Here's the drawing with two shaded views (mm, measured from the low corner). I have some questions. Coordinates: 2 decimals unless noted, no trailing zeros. Loops run counter-clockwise (first coordinate to the right, second up) from the corner with the lowest first, then second, coordinate; pieces in that order, holes last. Notation, with made-up numbers: M -12,-24.5 L 11,-24.5 A20 cw 11,3.5 Z; hole C 8.25,18.5 d2. An arc over 180 degrees is marked long. Return JSON: item names as keys, results as strings. Group by question number.
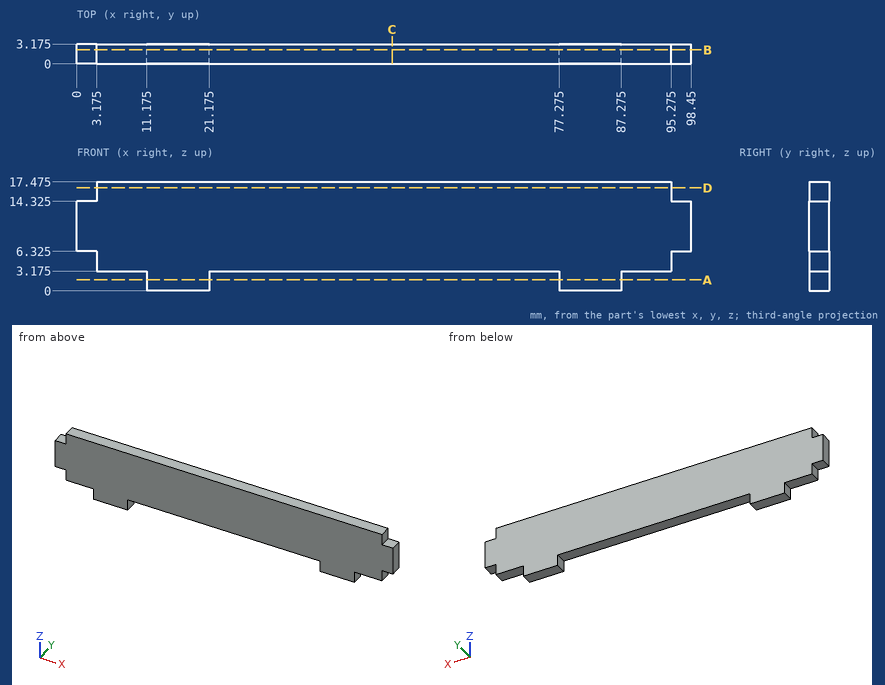
(1) Imagine slicing it at A-A, the plane z = 1.75. Write out the boundary of the cut face in (x, y) (3 decimals), then the cut area to 3 significant figures.
(2) Imagine slicing it at B-B, the plane y = 2.25. Write out the boundary of the cut face in (x, z) (3 decimals).
(3) Will these pins go through, and if not, where does the flat tip stop? P1, Ø1.6, axis at y = 1.5, z = 5, coming from the -X side (3 decimals); P2, Ø1, axis at y = 1, z = 1.5, coming from the +X side (3 decimals); P3, Ø1, axis at x = 69.5, y = 1, coming from the -Z side (3 decimals).
(4) Imagine slicing it at D-D, the plane z = 16.5. Write out the boundary of the cut face in (x, y) (3 decimals), then the cut area to 3 significant figures.
(5) If I drill on L1, parallel to X at y = 1.15, z = 2.25 (3 decimals); L2, parallel to Z at x = 71.5, y = 1.3 (3 decimals); L3, parallel to X at y = 1.65, z = 16 (3 decimals), over which ranges is the centre line in solid material (lowest first)? Write a range as [from, to].
(6) Imagine slicing it at C-C, the plane x = 50.5. Write out the boundary of the cut face in (y, z) (3 decimals).
Checks:
{
 "1": {"outline": "M 11.175,0 L 21.175,0 L 21.175,3.175 L 11.175,3.175 Z; M 77.275,0 L 87.275,0 L 87.275,3.175 L 77.275,3.175 Z", "area": "63.5 mm²"},
 "2": {"outline": "M 0,6.325 L 3.175,6.325 L 3.175,3.175 L 11.175,3.175 L 11.175,0 L 21.175,0 L 21.175,3.175 L 77.275,3.175 L 77.275,0 L 87.275,0 L 87.275,3.175 L 95.275,3.175 L 95.275,6.325 L 98.45,6.325 L 98.45,14.325 L 95.275,14.325 L 95.275,17.475 L 3.175,17.475 L 3.175,14.325 L 0,14.325 Z"},
 "3": {"P1": "x = 3.175", "P2": "x = 87.275", "P3": "z = 3.175"},
 "4": {"outline": "M 3.175,0 L 95.275,0 L 95.275,3.175 L 3.175,3.175 Z", "area": "292 mm²"},
 "5": {"L1": "[11.175, 21.175], [77.275, 87.275]", "L2": "[3.175, 17.475]", "L3": "[3.175, 95.275]"},
 "6": {"outline": "M 0,3.175 L 3.175,3.175 L 3.175,17.475 L 0,17.475 Z"}
}
